Autodesk Inventor part; units mm, degrees
ref_plane "YZ Plane" through (0, 0, 0) normal (1, 0, 0) x (0, 1, 0)
ref_plane "XZ Plane" through (0, 0, 0) normal (0, 1, 0) x (-1, 0, 0)
ref_plane "XY Plane" through (0, 0, 0) normal (0, 0, 1) x (1, 0, 0)
sketch "Sketch1" plane through (0, 0, 0) normal (0, 0, 1) x (1, 0, 0)
  arc A0 (0, 6.5) -> (0, -6.5) centre (0, 0) ccw
  line L0 (0, 6.5) -> (26, 6.5)
  line L1 (0, -6.5) -> (6.5, -6.5)
  arc A1 (26, -6.5) -> (26, 6.5) centre (26, 0) ccw
  line L2 (26, -6.5) -> (19.5, -6.5)
  line L3 (6.5, -6.5) -> (6.5, -45.5)
  line L4 (19.5, -6.5) -> (19.5, -45.5)
  line L5 (6.5, -45.5) -> (0, -45.5)
  arc A2 (0, -45.5) -> (0, -58.5) centre (0, -52) ccw
  line L6 (0, -58.5) -> (6.5, -58.5)
  arc A3 (6.5, -58.5) -> (19.5, -45.5) centre (6.5, -45.5) ccw
  line L7 (39, 0) -> (39, -52)
  arc A4 (39, -52) -> (52, -52) centre (45.5, -52) ccw
  line L8 (52, -52) -> (52, -32.5)
  line L9 (52, -32.5) -> (65, -32.5)
  line L10 (52, -6.5) -> (65, -6.5)
  line L11 (65, -6.5) -> (65, -19.5)
  line L12 (65, -19.5) -> (52, -19.5)
  line L13 (52, -19.5) -> (52, -6.5)
  line L14 (45.5, 6.5) -> (71.5, 6.5)
  line L15 (78, 0) -> (78, -52)
  line L16 (65, -32.5) -> (65, -52)
  arc A5 (65, -52) -> (78, -52) centre (71.5, -52) ccw
  arc A6 (45.5, 6.5) -> (39, 0) centre (45.5, 0) ccw
  arc A7 (78, 0) -> (71.5, 6.5) centre (71.5, 0) ccw
  line L17 (84.5, 0) -> (84.5, -26)
  arc A8 (91, 6.5) -> (84.5, 0) centre (91, 0) ccw
  line L18 (91, 6.5) -> (117, 6.5)
  line L19 (91, -32.5) -> (110.5, -32.5)
  arc A9 (84.5, -26) -> (91, -32.5) centre (91, -26) ccw
  line L20 (97.5, -6.5) -> (97.5, -19.5)
  line L21 (97.5, -6.5) -> (117, -6.5)
  arc A10 (117, -6.5) -> (117, 6.5) centre (117, 0) ccw
  line L22 (97.5, -19.5) -> (117, -19.5)
  arc A11 (123.5, -26) -> (117, -19.5) centre (117, -26) ccw
  line L23 (123.5, -26) -> (123.5, -52)
  line L24 (110.5, -32.5) -> (110.5, -45.5)
  line L25 (110.5, -45.5) -> (91, -45.5)
  arc A12 (91, -45.5) -> (91, -58.5) centre (91, -52) ccw
  arc A13 (117, -58.5) -> (123.5, -52) centre (117, -52) ccw
  line L26 (91, -58.5) -> (117, -58.5)
  line L27 (130, 0.001) -> (130, -51.999)
  line L28 (143, -6.499) -> (143, -45.499)
  line L29 (143, -6.499) -> (156, -6.499)
  line L30 (156, -6.499) -> (156, -45.499)
  line L31 (156, -45.499) -> (143, -45.499)
  arc A14 (136.5, 6.501) -> (130, 0.001) centre (136.5, 0.001) ccw
  line L32 (136.5, 6.501) -> (162.5, 6.501)
  line L33 (136.5, -58.499) -> (162.5, -58.499)
  arc A15 (162.5, -58.499) -> (169, -51.999) centre (162.5, -51.999) ccw
  line L34 (169, -51.999) -> (169, 0.001)
  arc A16 (169, 0.001) -> (162.5, 6.501) centre (162.5, 0.001) ccw
  line L35 (175.5, 0) -> (175.5, -52)
  arc A17 (175.524, -51.4421) -> (188.5, -52) centre (182, -52) ccw
  line L36 (214.5, -52.025) -> (214.5, 0.086)
  line L37 (188.5, -52) -> (188.5, -27.5463)
  line L38 (188.5, -27.5463) -> (202.1857, -54.9308)
  line L39 (201.5, 0.086) -> (201.5, -24.4787)
  line L40 (201.5, -24.4787) -> (187.8143, 2.9058)
  arc A18 (214.5, 0.086) -> (201.5, 0.086) centre (208, 0.086) ccw
  arc A19 (130, -51.9852) -> (136.5, -58.499) centre (136.5, -51.999) ccw
  arc A20 (202.1857, -54.9308) -> (214.5, -52.025) centre (208, -52.025) ccw
  arc A21 (187.8143, 2.9058) -> (175.5, 0) centre (182, 0) ccw
  point P0 (0, 0)
  dimension "d2" = 26
  dimension "d3" = 6.5
  dimension "d4" = 13
  dimension "d11" = 13
  dimension "d12" = 6.5
  dimension "d13" = 13
  dimension "d16" = 39
  dimension "d17" = 39
  dimension "d18" = 6.5
  dimension "d19" = 52
  dimension "d20" = 6.5
  dimension "d22" = 13
  dimension "d23" = 19.5
  dimension "d24" = 13
  dimension "d29" = 13
  dimension "d30" = 13
  dimension "d31" = 13
  dimension "d32" = 13
  dimension "d35" = 26
  dimension "d36" = 52
  dimension "d37" = 13
  dimension "d38" = 6.5
  dimension "d39" = 6.5
  dimension "d46" = 19.5
  dimension "d49" = 6.5
  dimension "d50" = 6.5
  dimension "d51" = 90
  dimension "d52" = 6.5
  dimension "d53" = 26
  dimension "d54" = 6.5
  dimension "d55" = 26
  dimension "d56" = 19.5
  dimension "d57" = 39
  dimension "d58" = 13
  dimension "d59" = 13
  dimension "d60" = 19.5
  dimension "d61" = 13
  dimension "d62" = 19.5
  dimension "d63" = 26
  dimension "d64" = 13
  dimension "d65" = 39
  dimension "d66" = 13
  dimension "d67" = 52
  dimension "d68" = 6.5
  dimension "d69" = 39
  dimension "d70" = 13
  dimension "d71" = 39
  dimension "d72" = 13
  dimension "d73" = 13
  dimension "d74" = 6.5
  dimension "d75" = 90
  dimension "d76" = 26
  dimension "d77" = 13
  dimension "d78" = 6.5
  dimension "d79" = 6.5
  dimension "d84" = 13
  dimension "d86" = 26
  dimension "d87" = 13
  dimension "d89" = 52
  dimension "d90" = 13
  dimension "d93" = 6.5
  dimension "d94" = 6.5
  dimension "d95" = 6.5
  dimension "d96" = 6.5
sketch "Sketch2" plane through (0, 0, 0) normal (0, 0, 1) x (1, 0, 0)
  circle A0 centre (231.3583, -77.1833) radius 3.175
  circle A1 centre (-20, 22) radius 3.175
  circle A2 centre (232, 22) radius 3.175
  circle A3 centre (-19.6417, -77.1833) radius 3.175
  line L0 (-29, 30) -> (240, 30)
  line L1 (240, 30) -> (240, -86)
  line L2 (240, -86) -> (-29, -86)
  line L3 (-29, -86) -> (-29, 30)
  point P0 (0, 0)
  dimension "d99" = 6.35
  dimension "d100" = 6.35
  dimension "d101" = 6.35
  dimension "d102" = 6.35
  dimension "d107" = 269
  dimension "d108" = 116
extrude "Extrusion1" add sketch "Sketch2" against normal blind 10
extrude "Extrusion2" cut sketch "Sketch1" against normal blind 5
properties part number "JASON" material "Polyethylene, High Density"
The model under review builds one solid part; all positions refer to its coordinate system, in mm. A direction names the side the tool comes from. Coordinates: 2 decimals unless noted, no trailing zeros. Write each loop counter-clockwise with the first axis right and the second up, starting at its lowest first coordinate (ties: lowest second). Pieces come first, ordered by that corner, then holes. Notation, with made-up numbers: (10, 88) - (41, 88) arc R15 cw to (41, 97) - close; hole circle Ø2 at (63, 43.25). An arc over 180 degrees is marked (long way). Answer in a Markdown table with one row per item. Add a question column.
Q1. Clearance check with flat-ended pins moving along their axes: pin 1 (8.5 mm diameter, centred on x = -19.64, y = -77.18, fed in from +Z); pin 2 (5.5 mm diameter, centred on x = 231.36, y = -77.18, fed in from +Z); pin 3 (4 mm diameter, centred on x = -0.5, y = 3.5, fed in from +Z). State where each tip first meets the part, or that it passes through.
Q2. Consider section C-C on x = 41.5. Give the boundary of the cut face in (y, z), then the cut area to 3 significant figures.
Q3. Consider section B-B on z = -3.5. Give the number of separate pieces and of enclosed holes in the cut face, then the cut area to 3 significant figures.
Q4. To check wall thickness, follow line 1 along X through (y, z) = (-77.5, -1.25); line 2 along Y through (x, z) = (232, -7.5) (3 decimals); line 3 along Y through (x, z) = (140, -3.5). State the ranges of each line that lie inside material, in increasing order. Write a range as from..to.
Q5. For faces 1 (the face through (-22.52, 20.07, -4.93)), 2 (the face through (110.5, -39, -2)), list the 3-axis set-ups (+Z, -Z, +X, -X, +Y, -Y) from which the entire face can be reached by the end or side of a thin tool; tool diameter is ignored.
Q6. Draft analysis for pull direction X (two halves, no side actions). For faces 3 (the face through (104, -40, 0)), 4 (the face through (-29, -29, -5)), 5 (the face through (97.5, -13, -2)), state which applies: +X half, -X half, draft (parallel to the pull), parting line (faces both ways), or undercut.
Q7. Consider section A-A on x = 208. Give the boundary of the cut face in (y, z), then the cut area to 3 significant figures.
Answers below:
| question | item | result |
|---|---|---|
| 1 | pin 1 | z = 0 |
| 1 | pin 2 | through |
| 1 | pin 3 | z = -5 |
| 2 | outline | (-86, -10) - (30, -10) - (30, 0) - (5.12, 0) - (5.12, -5) - (-57.12, -5) - (-57.12, 0) - (-86, 0) - close |
| 2 | area | 849 mm² |
| 3 | separate pieces | 3 |
| 3 | enclosed holes | 9 |
| 3 | area | 22,100 mm² |
| 4 | line 1 | -29..-22.8, -16.48..228.2, 234.52..240 |
| 4 | line 2 | -86..-80.293, -74.074..18.825, 25.175..30 |
| 4 | line 3 | -86..-58.5, 6.5..30 |
| 5 | face 1 | +Z, -Z |
| 5 | face 2 | +Z |
| 6 | face 3 | draft |
| 6 | face 4 | -X half |
| 6 | face 5 | undercut |
| 7 | outline | (-86, -10) - (30, -10) - (30, 0) - (6.59, 0) - (6.59, -5) - (-58.52, -5) - (-58.52, 0) - (-86, 0) - close |
| 7 | area | 834 mm² |
